Here's the drawing with two shaded views (mm, measured from the low corner). I have some questions. A direction names the side the tool comes from. Give positions to 0.01 mm unless a question says otherwise; leave off trailing zeros. Loops run counter-clockwise (first coordinate to the right, second up) from the corner with the lowest first, then second, coordinate; pieces in that order, holes last. Notation, with made-up numbers: (27.5, 42) - (80.5, 42) arc R15 ccw to (80.5, 69) - close; hole circle Ø2 at (26, -15.5). An arc over 180 degrees is marked (long way). Use a Markdown table: item, result. Add a question column.
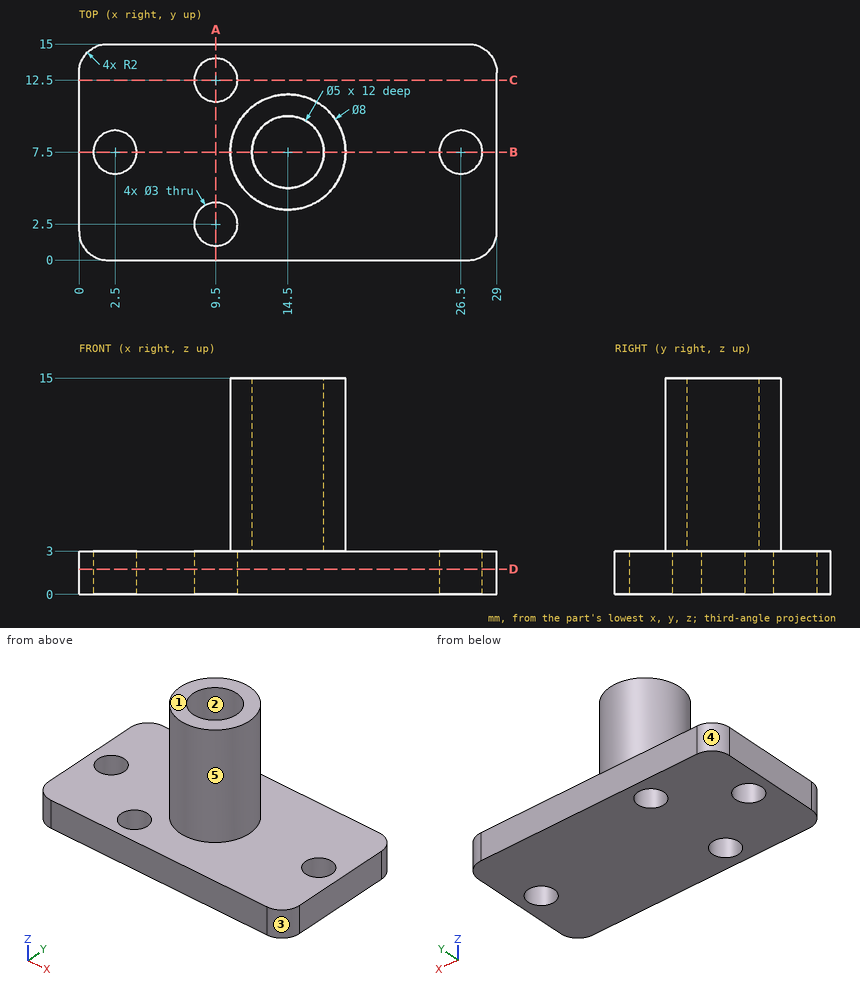
1. Suppose I cut it at D-D (z = 1.75). List the corners of the cut face in (x, y) for me, and give its area (3 significant figures).
2. On a 3-axis mill with a long thin cutter (end or side, diameter ignored), from which of +Z, -Z, +X, -X, +Y, -Y can I reach the whole of each face in a straight line? I mean the marked faces 4 and 5. Say none if no direction works.
3. Will these pins go through, and if not, where does the flat tip stop? P1, Ø4, axis at x = 9.5, y = 12.5, coming from the +Z side; P2, Ø1, axis at x = 12, z = 5.5, coming from the +Y side; P3, Ø6, axis at x = 15, z = 12, coming from the +Y side.
4. Suppose I cut it at B-B (y = 7.5). List the corners of the cut face in (x, z) for me, and give its area (3 significant figures).
5. If we mould it in two halves opening along X, with no side actions, what happens to the marked faces 1, 2 and 3? For each: released by +X, released by -X, zero draft, split by the parting line, or undercut.
6. Please list where these lines run through material, in increasing order: line 1 along Y through (x, z) = (9.5, 0.8); line 2 along Y through (x, z) = (2.5, 1.5); line 3 along X through (y, z) = (7.5, 6.5). Write a range as [from, to].
7. Suppose I cut it at C-C (y = 12.5). List the corners of the cut face in (x, z) for me, and give its area (3 significant figures).
8. Suppose I cut it at A-A (x = 9.5). List the corners of the cut face in (y, z) for me, and give its area (3 significant figures).
Results below:
| question | item | result |
|---|---|---|
| 1 | outline | (0, 2) arc R2 ccw to (2, 0) - (27, 0) arc R2 ccw to (29, 2) - (29, 13) arc R2 ccw to (27, 15) - (2, 15) arc R2 ccw to (0, 13) - close; hole circle Ø3 at (2.5, 7.5); hole circle Ø3 at (9.5, 2.5); hole circle Ø3 at (9.5, 12.5); hole circle Ø3 at (26.5, 7.5) |
| 1 | area | 403 mm² |
| 2 | face 4 | +Z, -Z, -X, +Y |
| 2 | face 5 | +Z |
| 3 | P1 | z = 3 |
| 3 | P2 | y = 10.96 |
| 3 | P3 | y = 11.5 |
| 4 | outline | (0, 0) - (1, 0) - (1, 3) - (0, 3) - close; (4, 0) - (25, 0) - (25, 3) - (18.5, 3) - (18.5, 15) - (17, 15) - (17, 3) - (12, 3) - (12, 15) - (10.5, 15) - (10.5, 3) - (4, 3) - close; (28, 0) - (29, 0) - (29, 3) - (28, 3) - close |
| 4 | area | 105 mm² |
| 5 | face 1 | zero draft |
| 5 | face 2 | undercut |
| 5 | face 3 | released by +X |
| 6 | line 1 | [0, 1], [4, 11], [14, 15] |
| 6 | line 2 | [0, 6], [9, 15] |
| 6 | line 3 | [10.5, 12], [17, 18.5] |
| 7 | outline | (0, 0) - (8, 0) - (8, 3) - (0, 3) - close; (11, 0) - (29, 0) - (29, 3) - (11, 3) - close |
| 7 | area | 78.0 mm² |
| 8 | outline | (0, 0) - (1, 0) - (1, 3) - (0, 3) - close; (4, 0) - (11, 0) - (11, 3) - (4, 3) - close; (14, 0) - (15, 0) - (15, 3) - (14, 3) - close |
| 8 | area | 27.0 mm² |
